from build123d import *

# Parameters (mm, degrees)
SKETCH1_W           = 1
SKETCH1_H           = 2.5
SKETCH1_W_2         = 10
SKETCH1_H_2         = 3.5
BOSS_EXTRUDE1_DEPTH = 1
BOSS_EXTRUDE2_START = 4.3
SKETCH1_3_W         = 1
SKETCH1_3_H         = 2.5
BOSS_EXTRUDE2_DEPTH = 4.3
CUT_EXTRUDE1_REACH  = 29.14
CUT_EXTRUDE2_DEPTH  = 33.393667716
BOSS_EXTRUDE4_START = 2
BOSS_EXTRUDE4_DEPTH = 2
SKETCH3_5_W         = 1
SKETCH3_5_H         = 0.8
BOSS_EXTRUDE5_DEPTH = 2.5
BOSS_EXTRUDE6_REACH = 31.992


with BuildPart() as part:
    # Sketch1 → Boss-Extrude1 (new body)
    # profile 1 of 4: a face of its own
    with BuildSketch(Plane(origin=(0, 0, 0), x_dir=(-1, 0, 0), z_dir=(0, 0, 1))):
        with BuildLine():
            ThreePointArc((-20.5, -7.1), (-21.914213562, -6.514213562), (-22.5, -5.1))
            Line((-22.5, -5.1), (-22.5, 4.115748324))
            ThreePointArc((-22.5, 4.115748324), (0, 15.804360023), (22.5, 4.115748324))
            Line((22.5, 4.115748324), (22.5, -5.1))
            ThreePointArc((22.5, -5.1), (21.914213562, -6.514213562), (20.5, -7.1))
            Line((20.5, -7.1), (-20.5, -7.1))
        make_face()
        with BuildLine():
            Line((-13, 6.5), (-13, 10.821020521))
            ThreePointArc((-13, 10.821020521), (0, 14.304360023), (13, 10.821020521))
            Line((13, 10.821020521), (13, 6.5))
            Line((13, 6.5), (17.2, 6.5))
            Line((17.2, 6.5), (17.2, 3))
            Line((17.2, 3), (19.5, 3))
            Line((19.5, 3), (19.5, -3))
            Line((19.5, -3), (17.2, -3))
            Line((17.2, -3), (17.2, -6.1))
            Line((17.2, -6.1), (-17.2, -6.1))
            Line((-17.2, -6.1), (-17.2, -3))
            Line((-17.2, -3), (-19.5, -3))
            Line((-19.5, -3), (-19.5, 3))
            Line((-19.5, 3), (-17.2, 3))
            Line((-17.2, 3), (-17.2, 6.5))
            Line((-17.2, 6.5), (-13, 6.5))
        make_face(mode=Mode.SUBTRACT)
    # profile 2 of 4: a face of its own
    with BuildSketch(Plane(origin=(0, 0, 0), x_dir=(-1, 0, 0), z_dir=(0, 0, 1))):
        with BuildLine():
            ThreePointArc((-13, 10.821020521), (0, 14.304360023), (13, 10.821020521))
            Line((13, 10.821020521), (13, 6.5))
            Line((13, 6.5), (17.2, 6.5))
            Line((17.2, 6.5), (17.2, 3))
            Line((17.2, 3), (19.5, 3))
            Line((19.5, 3), (19.5, -3))
            Line((19.5, -3), (17.2, -3))
            Line((17.2, -3), (17.2, -6.1))
            Line((17.2, -6.1), (-17.2, -6.1))
            Line((-17.2, -6.1), (-17.2, -3))
            Line((-17.2, -3), (-19.5, -3))
            Line((-19.5, -3), (-19.5, 3))
            Line((-19.5, 3), (-17.2, 3))
            Line((-17.2, 3), (-17.2, 6.5))
            Line((-17.2, 6.5), (-13, 6.5))
            Line((-13, 6.5), (-13, 10.821020521))
        make_face()
        with Locations((-18.2, 0)):
            Rectangle(SKETCH1_W, SKETCH1_H, mode=Mode.SUBTRACT)
        with Locations((0, 3.65)):
            Rectangle(SKETCH1_W_2, SKETCH1_H_2, mode=Mode.SUBTRACT)
        with Locations((18.2, 0)):
            Rectangle(SKETCH1_W, SKETCH1_H, mode=Mode.SUBTRACT)
    # profile 3 of 4: a face of its own
    with BuildSketch(Plane(origin=(0, 0, 0), x_dir=(-1, 0, 0), z_dir=(0, 0, 1))):
        with Locations((18.2, 0)):
            Rectangle(SKETCH1_W, SKETCH1_H)
    # profile 4 of 4: a face of its own
    with BuildSketch(Plane(origin=(0, 0, 0), x_dir=(-1, 0, 0), z_dir=(0, 0, 1))):
        with Locations((-18.2, 0)):
            Rectangle(SKETCH1_W, SKETCH1_H)
    extrude(amount=-BOSS_EXTRUDE1_DEPTH)

    # Sketch1<3> → Boss-Extrude2 (add)
    # profile 1 of 3: a face of its own
    with BuildSketch(Plane(origin=(0, 0, 0), x_dir=(-1, 0, 0), z_dir=(0, 0, 1)).offset(BOSS_EXTRUDE2_START)):
        with BuildLine():
            ThreePointArc((-20.5, -7.1), (-21.914213562, -6.514213562), (-22.5, -5.1))
            Line((-22.5, -5.1), (-22.5, 4.115748324))
            ThreePointArc((-22.5, 4.115748324), (0, 15.804360023), (22.5, 4.115748324))
            Line((22.5, 4.115748324), (22.5, -5.1))
            ThreePointArc((22.5, -5.1), (21.914213562, -6.514213562), (20.5, -7.1))
            Line((20.5, -7.1), (-20.5, -7.1))
        make_face()
        with BuildLine():
            Line((-13, 6.5), (-13, 10.821020521))
            ThreePointArc((-13, 10.821020521), (0, 14.304360023), (13, 10.821020521))
            Line((13, 10.821020521), (13, 6.5))
            Line((13, 6.5), (17.2, 6.5))
            Line((17.2, 6.5), (17.2, 3))
            Line((17.2, 3), (19.5, 3))
            Line((19.5, 3), (19.5, -3))
            Line((19.5, -3), (17.2, -3))
            Line((17.2, -3), (17.2, -6.1))
            Line((17.2, -6.1), (-17.2, -6.1))
            Line((-17.2, -6.1), (-17.2, -3))
            Line((-17.2, -3), (-19.5, -3))
            Line((-19.5, -3), (-19.5, 3))
            Line((-19.5, 3), (-17.2, 3))
            Line((-17.2, 3), (-17.2, 6.5))
            Line((-17.2, 6.5), (-13, 6.5))
        make_face(mode=Mode.SUBTRACT)
    # profile 2 of 3: a face of its own
    with BuildSketch(Plane(origin=(0, 0, 0), x_dir=(-1, 0, 0), z_dir=(0, 0, 1)).offset(BOSS_EXTRUDE2_START)):
        with Locations((18.2, 0)):
            Rectangle(SKETCH1_3_W, SKETCH1_3_H)
    # profile 3 of 3: a face of its own
    with BuildSketch(Plane(origin=(0, 0, 0), x_dir=(-1, 0, 0), z_dir=(0, 0, 1)).offset(BOSS_EXTRUDE2_START)):
        with Locations((-18.2, 0)):
            Rectangle(SKETCH1_3_W, SKETCH1_3_H)
    extrude(amount=-BOSS_EXTRUDE2_DEPTH)

    # Sketch3 → Cut-Extrude1 (cut, up to next)
    with BuildSketch(Plane.XZ.offset(1.25), mode=Mode.PRIVATE) as cut_extrude1_sk1:
        with BuildLine():
            Line((-17.7, 0), (-17.7, 1))
            ThreePointArc((-17.7, 1), (-17.833974596, 0.5), (-17.7, 0))
        make_face()
    cut_extrude1_tool1 = extrude(cut_extrude1_sk1.sketch, amount=-CUT_EXTRUDE1_REACH, mode=Mode.PRIVATE) & part.part
    # Sketch3 → Cut-Extrude1 (cut, up to next)
    with BuildSketch(Plane.XZ.offset(1.25), mode=Mode.PRIVATE) as cut_extrude1_sk2:
        with BuildLine():
            ThreePointArc((17.7, 0), (17.833974596, 0.5), (17.7, 1))
            Line((17.7, 1), (17.7, 0))
        make_face()
    cut_extrude1_tool2 = extrude(cut_extrude1_sk2.sketch, amount=-CUT_EXTRUDE1_REACH, mode=Mode.PRIVATE) & part.part
    add(cut_extrude1_tool1.solids().sort_by_distance((-17.75391, -1.25, 0.5))[0], mode=Mode.SUBTRACT)
    add(cut_extrude1_tool2.solids().sort_by_distance((17.75391, -1.25, 0.5))[0], mode=Mode.SUBTRACT)

    # Sketch4 → Cut-Extrude2 (cut, through all)
    with BuildSketch(Plane(origin=(0, 7.1, 0), x_dir=(1, 0, 0), z_dir=(0, 1, 0))):
        Polygon((19.5, 1), (19.5, -0.3), (22.5, -3.3), (22.5, 1), align=None)
        Polygon((-19.5, -0.3), (-22.5, -3.3), (-22.5, 1), (-19.5, 1), align=None)
    extrude(amount=-CUT_EXTRUDE2_DEPTH, mode=Mode.SUBTRACT)

    # Sketch5 → Boss-Extrude4 (add)
    with BuildSketch(Plane.XY.offset(4.3).offset(BOSS_EXTRUDE4_START)):
        with BuildLine():
            Line((17, -7.976675596), (17, -9.920326344))
            ThreePointArc((17, -9.920326344), (0, -15.804360023), (-17, -9.920326344))
            Line((-17, -9.920326344), (-17, -7.976675596))
            ThreePointArc((-17, -7.976675596), (0, -14.304360023), (17, -7.976675596))
        make_face()
    extrude(amount=-BOSS_EXTRUDE4_DEPTH)

    # Sketch3<5> → Boss-Extrude5 (add)
    with BuildSketch(Plane.XZ.offset(1.25)):
        with Locations((17.2, 2.4)):
            Rectangle(SKETCH3_5_W, SKETCH3_5_H)
        Polygon((16.7, 2), (17.7, 2), (17.7, 1), align=None)
        with Locations((-17.2, 2.4)):
            Rectangle(SKETCH3_5_W, SKETCH3_5_H)
        Polygon((-16.7, 2), (-17.7, 2), (-17.7, 1), align=None)
    extrude(amount=-BOSS_EXTRUDE5_DEPTH)

    # Sketch6 → Boss-Extrude6 (add, up to next)
    with BuildSketch(Plane.XZ.offset(-3), mode=Mode.PRIVATE) as boss_extrude6_sk1:
        Polygon((19.5, 2), (19.5, 0), (18.9, 0), align=None)
    boss_extrude6_tool1 = extrude(boss_extrude6_sk1.sketch, amount=BOSS_EXTRUDE6_REACH, mode=Mode.PRIVATE) - part.part
    # Sketch6 → Boss-Extrude6 (add, up to next)
    with BuildSketch(Plane.XZ.offset(-3), mode=Mode.PRIVATE) as boss_extrude6_sk2:
        Polygon((-18.9, 0), (-19.5, 2), (-19.5, 0), align=None)
    boss_extrude6_tool2 = extrude(boss_extrude6_sk2.sketch, amount=BOSS_EXTRUDE6_REACH, mode=Mode.PRIVATE) - part.part
    add(boss_extrude6_tool1.solids().sort_by_distance((19.3, 3, 0.666667))[0])
    add(boss_extrude6_tool2.solids().sort_by_distance((-19.3, 3, 0.666667))[0])


solid = part.part
Geometry check sheet. Reference: the model listing, model coordinates, mm. A direction names the side the tool comes from. Coordinates: 2 decimals unless noted, no trailing zeros. Loops run counter-clockwise (first coordinate to the right, second up) from the corner with the lowest first, then second, coordinate; pieces in that order, holes last. Notation, with made-up numbers: (-12.5, 65.5) - (20.5, 65.5) arc R23 cw to (20.5, 75.5) - close; hole circle Ø11 at (14, 82). An arc over 180 degrees is marked (long way). Use one line per item in the form item = value. Start each with the question number.
Item 1: Thickness scan on probe 1 along Y at (x, z) = (17, 4); probe 2 along X at (y, z) = (1.75, 4); probe 3 along X at (y, z) = (5.5, 0.25). Record the ranges inside material, lowest first.
Item 2: Tool access check on faces 3 (the face through (-18, 1.25, 2)), 4 (the face through (-17, -9, 5)), 5 (the face through (-17.834, -0.018, 0.507)). Record the directions out of +Z, -Z, +X, -X, +Y, -Y that give a thin tool (end or side, any length) a straight path to the whole face; none if there is none.
Item 3: Section check C-C, the plane x = -6. Enter the section's corners in (y, z), and give its area (3 significant figures).
Item 4: Mould release check, pull along Y, two halves, no side actions. Record for faces 1 (the face through (0, -15, 6.3)), 2 (the face through (-17.7, 0, 4)): +Y half, -Y half, draft (parallel to the pull), parting line (faces both ways), or undercut.
Item 5: Gauge pin test, flat ends, axial feed: pin 1 (6 mm diameter, centred on x = 6, y = -7.5, fed in from +Z); pin 2 (2 mm diameter, centred on y = -0.5, z = 1, fed in from -X); pin 3 (8 mm diameter, centred on x = -17.5, y = -3.5, fed in from +Z). Record the tip position at first contact, or that the pin passes through.
Item 6: Section check B-B, the plane x = -0.5. Enter the section's corners in (y, z), and give its area (3 significant figures).
Item 7: Section check A-A, the plane y = 3.75. Enter the section's corners in (x, z), and give its area (3 significant figures).
Computed:
q1.probe_1 = -9.92 to -6.5, 6.1 to 7.1
q1.probe_2 = -22.5 to -19.5, 19.5 to 22.5
q1.probe_3 = -19.5 to -17.2, 17.2 to 19.5
q2.face_3 = +Z
q2.face_4 = +Z, -X, +Y, -Y
q2.face_5 = none
q3.outline = (-15.14, -1) - (7.1, -1) - (7.1, 4.3) - (6.1, 4.3) - (6.1, 0) - (-13.6, 0) - (-13.6, 6.3) - (-15.14, 6.3) - close
q3.area = 36.2 mm2
q4.face_1 = draft
q4.face_2 = undercut
q5.pin_1 = 0
q5.pin_2 = -21.2
q5.pin_3 = 4.3
q6.outline = (-15.8, -1) - (-5.4, -1) - (-5.4, 0) - (-14.3, 0) - (-14.3, 6.3) - (-15.8, 6.3) - close; (-1.9, -1) - (7.1, -1) - (7.1, 4.3) - (6.1, 4.3) - (6.1, 0) - (-1.9, 0) - close
q6.area = 33.2 mm2
q7.outline = (-22.5, 3.3) - (-19.5, 0.3) - (-19.5, -1) - (19.5, -1) - (19.5, 0.3) - (22.5, 3.3) - (22.5, 4.3) - (17.2, 4.3) - (17.2, 0) - (-17.2, 0) - (-17.2, 4.3) - (-22.5, 4.3) - close
q7.area = 73.8 mm2
